Autodesk Inventor part; units mm, degrees
ref_plane "YZ Plane" through (0, 0, 0) normal (1, 0, 0) x (0, 1, 0)
ref_plane "XZ Plane" through (0, 0, 0) normal (0, 1, 0) x (-1, 0, 0)
ref_plane "XY Plane" through (0, 0, 0) normal (0, 0, 1) x (1, 0, 0)
sketch "Sketch1" plane through (0, 0, 0) normal (0, 1, 0) x (-1, 0, 0)
  point P0 (0, 0)
sketch "Sketch2" plane through (0, 0, 0) normal (0, 1, 0) x (-1, 0, 0)
  line L0 (0, 0) -> (62, 0)
  line L1 (62, 0) -> (62, -65)
  line L2 (62, -65) -> (0, -65)
  line L3 (0, -65) -> (0, 0)
  dimension "d0" = 62
  dimension "d1" = 65
extrude "Extrusion1" add sketch "Sketch2" along normal blind 12
sketch "Sketch3" plane through (0, 12, 0) normal (0, 1, 0) x (1, 0, 0)
  point P0 (0, 0)
sketch "Sketch4" plane through (0, 12, 0) normal (0, 1, 0) x (1, 0, 0)
  line L0 (0, 65) -> (-62, 65)
  line L1 (-30.4814, 65) -> (-28.4814, 65)
  line L2 (-28.4814, 65) -> (-28.4814, 63)
  line L3 (-62, 65) -> (-62, 0)
  line L4 (-62, 36.8423) -> (-62, 38.8423)
  line L5 (-62, 38.8423) -> (-60, 38.8423)
  line L6 (-62, 0) -> (0, 0)
  line L7 (-28.4814, 0) -> (-30.4814, 0)
  line L8 (-30.4814, 0) -> (-30.4814, 2)
  line L9 (0, 0) -> (0, 65)
  line L10 (0, 38.8423) -> (0, 36.8423)
  line L11 (0, 36.8423) -> (-2, 36.8423)
  line L12 (-60, 63) -> (-2, 63)
  line L13 (-2, 63) -> (-2, 2)
  line L14 (-2, 2) -> (-60, 2)
  line L15 (-60, 2) -> (-60, 63)
  dimension "d5" = 2
  dimension "d6" = 2
  dimension "d7" = 2
  dimension "d8" = 2
  dimension "d9" = 2
  dimension "d10" = 2
  dimension "d11" = 2
  dimension "d12" = 2
extrude "Extrusion2" cut sketch "Sketch4" against normal blind 10 contours L12 L13 L14 L15
sketch "Sketch10" plane through (0, 2, 0) normal (0, 1, 0) x (1, 0, 0)
  line L0 (-2, 2) -> (-60, 2)
  line L1 (-31, 2) -> (-41, 2)
  line L2 (-41, 2) -> (-41, 4)
  line L3 (-41, 2) -> (-51, 2)
  line L4 (-51, 2) -> (-51, 4)
  line L5 (-51, 4) -> (-41, 4)
  line L6 (-41, 4) -> (-41, 2)
  line L7 (-60, 63) -> (-2, 63)
  line L8 (-51, 63) -> (-41, 63)
  line L9 (-41, 63) -> (-41, 61)
  line L10 (-41, 61) -> (-51, 61)
  line L11 (-51, 61) -> (-51, 63)
  line L12 (-60, 2) -> (-60, 63)
  line L13 (-21, 63) -> (-11, 63)
  line L14 (-11, 63) -> (-11, 61)
  line L15 (-11, 61) -> (-21, 61)
  line L16 (-21, 61) -> (-21, 63)
  line L17 (-21, 2) -> (-11, 2)
  line L18 (-11, 2) -> (-11, 4)
  line L19 (-11, 4) -> (-21, 4)
  line L20 (-21, 4) -> (-21, 2)
  line L21 (-2, 63) -> (-2, 2)
  point P0 (0, 0)
  dimension "d55" = 2
  dimension "d56" = 10
  dimension "d57" = 10
  dimension "d58" = 2
  dimension "d59" = 9
  dimension "d60" = 10
  dimension "d61" = 10
  dimension "d62" = 9
  dimension "d63" = 9
extrude "Extrusion5" add sketch "Sketch10" along normal blind 9 contours L0 L20 L19 L18 | L14 L15 L16 L7 | L0 L4 L5 L2 | L9 L10 L11 L7
sketch "Sketch12" plane through (0, 0, 0) normal (0, -1, 0) x (1, 0, 0)
  line L0 (0, 0) -> (0, -65)
  arc A0 (-33, -49.3087) -> (-29, -49.3087) centre (-31, -51.5448) ccw
  arc A1 (-29, -46.2034) -> (-33, -46.2034) centre (-31, -46.2034) ccw
  line L1 (-29, -46.2034) -> (-29, -49.3087)
  line L2 (-33, -46.2034) -> (-33, -49.3087)
extrude "Extrusion7" cut sketch "Sketch12" against normal blind 10
sketch "Sketch13" plane through (0, 12, 0) normal (0, 1, 0) x (1, 0, 0)
  line L0 (-60, 2) -> (-60, 63)
  line L1 (-60, 4.6965) -> (-61, 4.6965)
  line L2 (-62, 65) -> (-62, 0)
  line L3 (-55.851, 2) -> (-55.851, 1)
  line L4 (-2, 63) -> (-2, 2)
  line L5 (-2, 53.5974) -> (-2, 54.5974)
  line L6 (-2, 54.5974) -> (-1, 54.5974)
  line L7 (0, 0) -> (0, 65)
  line L8 (-60, 63) -> (-2, 63)
  line L9 (-54.9589, 63) -> (-55.9589, 63)
  line L10 (-55.9589, 63) -> (-56.9589, 63)
  line L11 (-56.9589, 63) -> (-56.9589, 64)
  line L12 (-61, 1) -> (-1, 1)
  line L13 (-1, 1) -> (-1, 64)
  line L14 (-1, 64) -> (-61, 64)
  line L15 (-61, 64) -> (-61, 1)
  dimension "d81" = 1
  dimension "d82" = 1
  dimension "d83" = 1
  dimension "d84" = 1
  dimension "d85" = 1
  dimension "d86" = 1
  dimension "d87" = 1
extrude "Extrusion8" cut sketch "Sketch13" against normal blind 2
properties part number "Shell 1"
Source: CAD feature listing. Evaluate the final solid. Frame: model axes, mm. A direction names the side the tool comes from. Coordinates: 2 decimals unless noted, no trailing zeros. Loops run counter-clockwise (first coordinate to the right, second up) from the corner with the lowest first, then second, coordinate; pieces in that order, holes last. Notation, with made-up numbers: M -21.75,51 L -15.75,51 A32 ccw -15.75,86 Z; hole C 0.5,30.25 d7. An arc over 180 degrees is marked long. Put each result on its own line as item: value. Start each with the question number.
1) Ray query, L1, parallel to Z at x = -31, y = 0.75; L2, parallel to X at y = 3, z = -40.5; L3, parallel to X at y = 11, z = -56. Return the intervals inside material, ascending. Write a range as from..to.
2) Cut plane B-B on y = 8. Return the cut outline in (x, z).
3) Contact query for a flat-ended pin moving along its axis: pin 1 Ø6 at (x, z) = (-18, -51.5) entering from +Y. Output: stop coordinate, or through.
4) Cut plane D-D on x = -23.5. Return the cut outline in (y, z).
5) Cut plane A-A on x = -31. Return the cut outline in (y, z), then the cut area to 3 significant figures.
6) Pull-direction query (Z, two-part tool) for faces 3 (the face through (-62, 6, -32)), 4 (the face through (-31, 6, -65)), 5 (the face through (-11, 6, -3)); classes: pulls with the +Z half, pulls with the -Z half, needs draft (parallel to the pull), parting line crosses it, or undercut.
7) Cut plane C-C on z = -53. Return the cut outline in (x, y).
8) Reachability of faces 1 (the face through (-29, 1, -48)), 2 (the face through (-21, 6, -62)) from +Z, -Z, +X, -X, +Y, -Y: full face, straight path, thin tool, end or side. Return the list, or none.
The answers:
1. L1: z = -65..-54.54, -44.2..0
1. L2: x = -62..-60, -2..0
1. L3: x = -62..-61, -1..0
2. outline: M -62,-65 L 0,-65 L 0,0 L -62,0 Z; hole M -60,-63 L -51,-63 L -51,-61 L -41,-61 L -41,-63 L -21,-63 L -21,-61 L -11,-61 L -11,-63 L -2,-63 L -2,-2 L -11,-2 L -11,-4 L -21,-4 L -21,-2 L -41,-2 L -41,-4 L -51,-4 L -51,-2 L -60,-2 Z
3. pin 1: stops at y = 2
4. outline: M 0,-65 L 12,-65 L 12,-64 L 10,-64 L 10,-63 L 2,-63 L 2,-2 L 10,-2 L 10,-1 L 12,-1 L 12,0 L 0,0 Z
5. outline: M 0,-65 L 12,-65 L 12,-64 L 10,-64 L 10,-63 L 2,-63 L 2,-54.54 L 0,-54.54 Z; M 0,-44.2 L 2,-44.2 L 2,-2 L 10,-2 L 10,-1 L 12,-1 L 12,0 L 0,0 Z
5. area: 145 mm²
6. face 3: needs draft
6. face 4: pulls with the -Z half
6. face 5: undercut
7. outline: M -62,0 L -33.62,0 L -33.62,2 L -60,2 L -60,10 L -61,10 L -61,12 L -62,12 Z; M -28.38,0 L 0,0 L 0,12 L -1,12 L -1,10 L -2,10 L -2,2 L -28.38,2 Z
8. face 1: +Y, -Y
8. face 2: +Y
